Design review of the part built by this model. Coordinates are the model's own, in mm. A direction names the side the tool comes from. Coordinates: 2 decimals unless noted, no trailing zeros. Write each loop counter-clockwise with the first axis right and the second up, starting at its lowest first coordinate (ties: lowest second). Pieces come first, ordered by that corner, then holes. Notation, with made-up numbers: (-15.75, -20.75) - (36.25, -20.75) arc R11 ccw to (36.25, -1.75) - close; hole circle Ø7 at (57.25, -18). An arc over 180 degrees is marked (long way). Use a Markdown table: item, result.
from build123d import *

# Parameters (mm, degrees)
ESQUISSE1_W        = 5
ESQUISSE1_H        = 5
BOSS_EXTRU_1_DEPTH = 5


with BuildPart() as part:
    # Esquisse1 → Boss.-Extru.1 (new body)
    with BuildSketch(Plane.XY):
        with BuildLine():
            Line((0, 0), (-5, 0))
            Line((-5, 0), (-5, -5))
            Line((-5, -5), (-10, -5))
            Line((-10, -5), (-10, 0))
            Line((-10, 0), (-13.5, 0))
            Line((-13.5, 0), (-13.5, 3))
            Line((-13.5, 3), (-12.4, 3))
            Line((-12.4, 3), (-12.4, 5.3))
            Line((-12.4, 5.3), (-13.5, 5.3))
            Line((-13.5, 5.3), (-13.5, 10))
            Line((-13.5, 10), (-16.5, 10))
            Line((-16.5, 10), (-16.5, 5.3))
            Line((-16.5, 5.3), (-17.6, 5.3))
            Line((-17.6, 5.3), (-17.6, 3))
            Line((-17.6, 3), (-16.5, 3))
            Line((-16.5, 3), (-16.5, 0))
            Line((-16.5, 0), (-20, 0))
            Line((-20, 0), (-20, -5))
            Line((-20, -5), (-25, -5))
            Line((-25, -5), (-25, 0))
            Line((-25, 0), (-30, 0))
            Line((-30, 0), (-30, 13.133014138))
            ThreePointArc((-30, 13.133014138), (-30.275608697, 14.274102799), (-31.041666667, 15.163596293))
            ThreePointArc((-31.041666667, 15.163596293), (-42.5, 37.5), (-31.041666667, 59.836403707))
            ThreePointArc((-31.041666667, 59.836403707), (-30.275608697, 60.725897201), (-30, 61.866985862))
            Line((-30, 61.866985862), (-30, 75))
            Line((-30, 75), (-25, 75))
            Line((-25, 75), (-25, 80))
            Line((-25, 80), (-20, 80))
            Line((-20, 80), (-20, 75))
            Line((-20, 75), (-16.5, 75))
            Line((-16.5, 75), (-16.5, 72))
            Line((-16.5, 72), (-17.6, 72))
            Line((-17.6, 72), (-17.6, 69.7))
            Line((-17.6, 69.7), (-16.5, 69.7))
            Line((-16.5, 69.7), (-16.5, 65))
            Line((-16.5, 65), (-13.5, 65))
            Line((-13.5, 65), (-13.5, 69.7))
            Line((-13.5, 69.7), (-12.4, 69.7))
            Line((-12.4, 69.7), (-12.4, 72))
            Line((-12.4, 72), (-13.5, 72))
            Line((-13.5, 72), (-13.5, 75))
            Line((-13.5, 75), (-10, 75))
            Line((-10, 75), (-10, 80))
            Line((-10, 80), (-5, 80))
            Line((-5, 80), (-5, 75))
            Line((-5, 75), (0, 75))
            Line((0, 75), (0, 61.866985862))
            ThreePointArc((0, 61.866985862), (0.275608697, 60.725897201), (1.041666667, 59.836403707))
            ThreePointArc((1.041666667, 59.836403707), (8.082814572, 52.447697864), (11.944387171, 43))
            ThreePointArc((11.944387171, 43), (11.431389101, 40.91886117), (9.494897428, 40))
            Line((9.494897428, 40), (2.827296486, 40))
            ThreePointArc((2.827296486, 40), (-0.374759815, 40.92586604), (-2.588591054, 43.417721519))
            ThreePointArc((-2.588591054, 43.417721519), (-28.75, 37.5), (-2.588591054, 31.582278481))
            ThreePointArc((-2.588591054, 31.582278481), (-0.374759815, 34.07413396), (2.827296486, 35))
            Line((2.827296486, 35), (9.494897428, 35))
            ThreePointArc((9.494897428, 35), (11.431389101, 34.08113883), (11.944387171, 32))
            ThreePointArc((11.944387171, 32), (8.082814572, 22.552302136), (1.041666667, 15.163596293))
            ThreePointArc((1.041666667, 15.163596293), (0.275608697, 14.274102799), (0, 13.133014138))
            Line((0, 13.133014138), (0, 0))
        make_face()
        with Locations((-15, 57.9)):
            Rectangle(ESQUISSE1_W, ESQUISSE1_H, mode=Mode.SUBTRACT)
        Polygon((3.581981747, 51.115063509), (6.081981747, 46.784936491), (1.751854728, 44.284936491), (-0.748145272, 48.615063509), align=None, mode=Mode.SUBTRACT)
        Polygon((6.081981747, 28.215063509), (3.581981747, 23.884936491), (-0.748145272, 26.384936491), (1.751854728, 30.715063509), align=None, mode=Mode.SUBTRACT)
        with Locations((-15, 17.1)):
            Rectangle(ESQUISSE1_W, ESQUISSE1_H, mode=Mode.SUBTRACT)
        Polygon((-33.581981747, 23.884936491), (-36.081981747, 28.215063509), (-31.751854728, 30.715063509), (-29.251854728, 26.384936491), align=None, mode=Mode.SUBTRACT)
        Polygon((-36.081981747, 46.784936491), (-33.581981747, 51.115063509), (-29.251854728, 48.615063509), (-31.751854728, 44.284936491), align=None, mode=Mode.SUBTRACT)
    extrude(amount=BOSS_EXTRU_1_DEPTH)


solid = part.part
(1) Take a section at A-A on x = -26. Write out the cut boundary in (y, z).
Determined:
| item | result |
|---|---|
| outline | (0, 0) - (29.25, 0) - (29.25, 5) - (0, 5) - close; (45.75, 0) - (75, 0) - (75, 5) - (45.75, 5) - close |
(2) For pin 1 (6 mm diameter, centred on x = -29, y = 24.5, fed in from -Z); pin 2 (2.5 mm diameter, centred on y = 73, z = 3, fed in from +X); pin 3 (1 mm diameter, centred on x = 4, z = 1.5, fed in from +Y); pin 4 (1.5 mm diameter, centred on x = -15, z = 2.5, fed in from +Y), all flat-tipped, find the tip position at first contact; note any pin that passes through.
Determined:
| item | result |
|---|---|
| pin 1 | z = 0 |
| pin 2 | x = 0 |
| pin 3 | y = 57.85 |
| pin 4 | y = 65 |
(3) Take a section at D-D on z = 2.9. State how many separate pieces and enclosed holes the cut face has, and give its area (3 significant figures).
Determined:
| item | result |
|---|---|
| separate pieces | 1 |
| enclosed holes | 6 |
| area | 2,270 mm2 |
(4) Machinability: for faces 5 (the flat face through (-16.5, 67, 2)), 6 (the flat face through (6, 40, 2)), 7 (the flat face through (-5, -2, 2)), 8 (the flat face through (-12.4, 71, 2)), which of the approach directions +Z, -Z, +X, -X, +Y, -Y give a long, thin tool a straight path to every point of the face, cutting with its end or side? Answer none if there is none.
Determined:
| item | result |
|---|---|
| face 5 | +Z, -Z, +Y |
| face 6 | +Z, -Z, +X |
| face 7 | +Z, -Z, +X, -Y |
| face 8 | +Z, -Z |
(5) Take a section at C-C on x = 5. Write out the cut boundary in (y, z), and give its area (3 significant figures).
Determined:
| item | result |
|---|---|
| outline | (18.63, 0) - (26.34, 0) - (26.34, 5) - (18.63, 5) - close; (28.84, 0) - (35, 0) - (35, 5) - (28.84, 5) - close; (40, 0) - (46.16, 0) - (46.16, 5) - (40, 5) - close; (48.66, 0) - (56.37, 0) - (56.37, 5) - (48.66, 5) - close |
| area | 139 mm2 |
(6) Take a section at B-B on y = 66. Write out the cut boundary in (x, z).
Determined:
| item | result |
|---|---|
| outline | (-30, 0) - (-16.5, 0) - (-16.5, 5) - (-30, 5) - close; (-13.5, 0) - (0, 0) - (0, 5) - (-13.5, 5) - close |
(7) Draft analysis for pull direction X (two halves, no side actions). For faces 1 (the flat face through (-33.89, 45.52, 2.46)), 2 (the flat face through (-12, 0, 2)), 3 (the cylindrical face through (11.41, 34.11, 2.46)), 4 (the flat face through (-22, -5, 2)), state which applies: +X half, -X half, draft (parallel to the pull), parting line (faces both ways), or undercut.
Determined:
| item | result |
|---|---|
| face 1 | undercut |
| face 2 | undercut |
| face 3 | +X half |
| face 4 | draft |
(8) For L1, parallel to Y at x = -15, z = 3.8; L2, parallel to X at y = 8, z = 1.45; L3, parallel to X at y = 25, z = 4.1, list the stretches that pass through material, from the lowest coordinate up. Write a range as from..to.
Determined:
| item | result |
|---|---|
| L1 | 10..14.6, 19.6..23.75, 51.25..55.4, 60.4..65 |
| L2 | -30..-16.5, -13.5..0 |
| L3 | -39.49..-34.23, -31.65..-20.73, -9.27..1.65, 4.23..9.49 |
